from build123d import *

# Parameters (mm, degrees)
SKETCH1_R                = 150
BOSS_EXTRUDE1_DEPTH      = 75
CHAMFER1_SIZE            = 10
BOSS_EXTRUDE2_START      = -75
BOSS_EXTRUDE2_DEPTH      = 10
CHAMFER2_SIZE            = 10
BOSS_EXTRUDE3_DEPTH      = 10
BOSS_EXTRUDE4_DEPTH      = 3.5
CIRPATTERN1_COUNT        = 4
CIRPATTERN1_COPY_1_DEPTH = 10
CIRPATTERN1_COPY_2_DEPTH = 10
CIRPATTERN1_COPY_3_DEPTH = 10
CIRPATTERN1_COPY_4_DEPTH = 3.5
CIRPATTERN1_COPY_5_DEPTH = 3.5
CIRPATTERN1_COPY_6_DEPTH = 3.5
CUT_EXTRUDE1_START       = -50
CUT_EXTRUDE1_DEPTH       = 50
CIRPATTERN2_COUNT        = 4
SKETCH7_R                = 110
BOSS_EXTRUDE5_DEPTH      = 9
BOSS_EXTRUDE5_TAPER      = 45
SKETCH8_R                = 15
BOSS_EXTRUDE6_DEPTH      = 20
SKETCH9_W                = 52.192884268
SKETCH9_H                = 17.88463766
BOSS_EXTRUDE7_DEPTH      = 3
BOSS_EXTRUDE8_DEPTH      = 2


# Read off the part's stored shape, not the designer's step: Cut-Extrude1
with BuildPart() as part:
    # Sketch1 → Boss-Extrude1 (new body)
    with BuildSketch(Plane(origin=(0, 0, 0), x_dir=(1, 0, 0), z_dir=(0, 1, 0))):
        with Locations(Location((0, 0, 0), (0, 0, 270))):
            Circle(SKETCH1_R)
    extrude(amount=BOSS_EXTRUDE1_DEPTH)

    # Chamfer1
    chamfer1_edges = [part.edges().sort_by_distance(p)[0] for p in [
        (0, 75, -150),
    ]]
    chamfer(chamfer1_edges, length=CHAMFER1_SIZE)

    # Sketch3 → Boss-Extrude2 (add)
    with BuildSketch(Plane(origin=(0, 75, 0), x_dir=(1, 0, 0), z_dir=(0, 1, 0)).offset(BOSS_EXTRUDE2_START)):
        with BuildLine():
            Line((-145.236875483, 37.5), (-195.236875483, 37.5))
            Line((-195.236875483, 37.5), (-195.236875483, -37.5))
            Line((-195.236875483, -37.5), (-145.236875483, -37.5))
            ThreePointArc((-145.236875483, -37.5), (-150, 0), (-145.236875483, 37.5))
        make_face()
    boss_extrude2 = extrude(amount=BOSS_EXTRUDE2_DEPTH)

    # Chamfer2
    chamfer2_edges = [part.edges().sort_by_distance(p)[0] for p in [
        (-195.236875483, 5, -37.5),
        (-195.236875483, 5, 37.5),
    ]]
    chamfer(chamfer2_edges, length=CHAMFER2_SIZE)

    # Sketch4 → Boss-Extrude3 (add)
    with BuildSketch(Plane.XY.offset(37.5)):
        Polygon((-185.236875483, 10), (-145.236875483, 10), (-145.236875483, 65), (-168.236875483, 65), align=None)
    boss_extrude3 = extrude(amount=-BOSS_EXTRUDE3_DEPTH)

    # Sketch5 → Boss-Extrude4 (add)
    with BuildSketch(Plane(origin=(0, 10, 0), x_dir=(1, 0, 0), z_dir=(0, 1, 0))):
        Polygon((-185.236875483, -20), (-180.04072306, -17), (-180.04072306, -11), (-185.236875483, -8), (-190.433027905, -11), (-190.433027905, -17), align=None)
    boss_extrude4 = extrude(amount=BOSS_EXTRUDE4_DEPTH)

    # Mirror1: Boss-Extrude3, Boss-Extrude4 across plane
    add(boss_extrude3.mirror(Plane.XY))
    add(boss_extrude4.mirror(Plane.XY))

    # CirPattern1: Boss-Extrude2, Boss-Extrude3, Boss-Extrude4 ×4 about axis
    cirpattern1_axis = Axis((0, 0, 0), (0, 1, 0))
    add([boss_extrude2.rotate(cirpattern1_axis, i * 360 / CIRPATTERN1_COUNT) for i in range(1, CIRPATTERN1_COUNT)])
    add([boss_extrude3.rotate(cirpattern1_axis, i * 360 / CIRPATTERN1_COUNT) for i in range(1, CIRPATTERN1_COUNT)])
    add([boss_extrude4.rotate(cirpattern1_axis, i * 360 / CIRPATTERN1_COUNT) for i in range(1, CIRPATTERN1_COUNT)])

    # CirPattern1 copy 1 sketch → CirPattern1 copy 1 (add)
    with BuildSketch(Plane(origin=(-37.5, 0, 0), x_dir=(0, 0, -1), z_dir=(-1, 0, 0))):
        Polygon((-185.236875483, -10), (-145.236875483, -10), (-145.236875483, -65), (-168.236875483, -65), align=None)
    extrude(amount=-CIRPATTERN1_COPY_1_DEPTH)

    # CirPattern1 copy 2 sketch → CirPattern1 copy 2 (add)
    with BuildSketch(Plane(origin=(0, 0, 37.5), x_dir=(-1, 0, 0), z_dir=(0, 0, 1))):
        Polygon((-185.236875483, -10), (-145.236875483, -10), (-145.236875483, -65), (-168.236875483, -65), align=None)
    extrude(amount=-CIRPATTERN1_COPY_2_DEPTH)

    # CirPattern1 copy 3 sketch → CirPattern1 copy 3 (add)
    with BuildSketch(Plane(origin=(37.5, 0, 0), x_dir=(0, 0, 1), z_dir=(1, 0, 0))):
        Polygon((-185.236875483, -10), (-145.236875483, -10), (-145.236875483, -65), (-168.236875483, -65), align=None)
    extrude(amount=-CIRPATTERN1_COPY_3_DEPTH)

    # CirPattern1 copy 4 sketch → CirPattern1 copy 4 (add)
    with BuildSketch(Plane(origin=(0, 10, 0), x_dir=(0, 0, -1), z_dir=(0, 1, 0))):
        Polygon((-185.236875483, 20), (-180.04072306, 17), (-180.04072306, 11), (-185.236875483, 8), (-190.433027905, 11), (-190.433027905, 17), align=None)
    extrude(amount=CIRPATTERN1_COPY_4_DEPTH)

    # CirPattern1 copy 5 sketch → CirPattern1 copy 5 (add)
    with BuildSketch(Plane(origin=(0, 10, 0), x_dir=(-1, 0, 0), z_dir=(0, 1, 0))):
        Polygon((-185.236875483, 20), (-180.04072306, 17), (-180.04072306, 11), (-185.236875483, 8), (-190.433027905, 11), (-190.433027905, 17), align=None)
    extrude(amount=CIRPATTERN1_COPY_5_DEPTH)

    # CirPattern1 copy 6 sketch → CirPattern1 copy 6 (add)
    with BuildSketch(Plane.ZX.offset(10)):
        Polygon((-185.236875483, 20), (-180.04072306, 17), (-180.04072306, 11), (-185.236875483, 8), (-190.433027905, 11), (-190.433027905, 17), align=None)
    extrude(amount=CIRPATTERN1_COPY_6_DEPTH)

    # Cut-Extrude1 outline → Cut-Extrude1 (cut)
    with BuildSketch(Plane(origin=(0, 75, 0), x_dir=(1, 0, 0), z_dir=(0, 1, 0)).offset(CUT_EXTRUDE1_START)):
        with BuildLine():
            ThreePointArc((-65, -112.583302492), (-91.923881554, -91.923881554), (-112.583302492, -65))
            Line((-112.583302492, -65), (-129.903810568, -75))
            ThreePointArc((-129.903810568, -75), (-106.066017178, -106.066017178), (-75, -129.903810568))
            Line((-75, -129.903810568), (-65, -112.583302492))
        make_face()
    cut_extrude1 = extrude(amount=CUT_EXTRUDE1_DEPTH, mode=Mode.SUBTRACT)

    # CirPattern2: Cut-Extrude1 ×4 about axis
    cirpattern2_axis = Axis((1.096442134, 0, -1.096442134), (0, 1, 0))
    for i in range(1, CIRPATTERN2_COUNT):
        add(cut_extrude1.rotate(cirpattern2_axis, i * 360 / CIRPATTERN2_COUNT), mode=Mode.SUBTRACT)

    # Sketch7 → Boss-Extrude5 (add)
    with BuildSketch(Plane(origin=(0, 75, 0), x_dir=(1, 0, 0), z_dir=(0, 1, 0))):
        Circle(SKETCH7_R)
    extrude(amount=BOSS_EXTRUDE5_DEPTH, taper=BOSS_EXTRUDE5_TAPER)

    # Sketch8 → Boss-Extrude6 (add)
    with BuildSketch(Plane(origin=(0, 84, 0), x_dir=(1, 0, 0), z_dir=(0, 1, 0))):
        with Locations(Location((0, 0, 0), (0, 0, 270))):
            Circle(SKETCH8_R)
    extrude(amount=BOSS_EXTRUDE6_DEPTH)

    # Sketch9 → Boss-Extrude7 (add)
    with BuildSketch(Plane(origin=(0, 75, 0), x_dir=(1, 0, 0), z_dir=(0, 1, 0))):
        with Locations((1.096442134, -121.525621322)):
            Rectangle(SKETCH9_W, SKETCH9_H)
    extrude(amount=BOSS_EXTRUDE7_DEPTH)

    # Sketch10 → Boss-Extrude8 (add)
    with BuildSketch(Plane(origin=(0, 78, 0), x_dir=(1, 0, 0), z_dir=(0, 1, 0))):
        with BuildLine():
            Line((6.270682812, -126.545342988), (8.874678556, -128.884668308))
            Line((8.874678556, -128.884668308), (10.207504523, -127.401046891))
            Line((10.207504523, -127.401046891), (7.367027593, -124.84927636))
            ThreePointArc((7.367027593, -124.84927636), (-4.827336948, -118.169160855), (6.270682812, -126.545342988))
        make_face()
        with BuildLine():
            Line((4.310616526, -122.103519263), (2.977790559, -123.58714068))
            Line((2.977790559, -123.58714068), (4.010713475, -124.515077192))
            ThreePointArc((4.010713475, -124.515077192), (-2.528998008, -120.272284372), (4.900321371, -122.63328644))
            Line((4.900321371, -122.63328644), (4.310616526, -122.103519263))
        make_face(mode=Mode.SUBTRACT)
    extrude(amount=BOSS_EXTRUDE8_DEPTH)


solid = part.part
For this review, take the finished solid that the model builds, in its own axes (mm). A direction names the side the tool comes from. Coordinates: 2 decimals unless noted, no trailing zeros. Order: outer loops, then holes, each group sorted by start corner. A loop starts at its lowest first (then second) coordinate and runs counter-clockwise, first axis right, second up. Notation, with made-up numbers: (-35.75, -8) - (3.25, -8) arc R33 cw to (3.25, 24) - close; hole circle Ø3 at (18.5, -1.5). An arc over 180 degrees is marked (long way). Answer as CSV lines item,"result". Start each with the question number.
1) Insertion check: P1, Ø8, axis at x = 56.5, z = -34.5, coming from the +Y side; P2, Ø1, axis at x = 76.5, y = 57, coming from the -Z side; P3, Ø6, axis at y = 17.5, z = -124.5, coming from the +X side. Each pin has a flat end and moves straight along its axis. Give the tip position at first contact, or say it passes through.
2) Machinability: for faces 1 (the flat face through (185, 13.5, 14)), 2 (the flat face through (14, 13.5, 185)), 3 (the flat face through (-161, 33, -37.5)), 4 (the flat face through (33, 65, -157)), which of the approach directions +Z, -Z, +X, -X, +Y, -Y give a long, thin tool a straight path to every point of the face, cutting with its end or side? Answer none if there is none.
3) To check wall thickness, follow line 1 along Z through (x, y) = (10.5, 12); line 2 along Y through (x, z) = (-112.5, -78.5); line 3 along Z through (x, y) = (-153, 26.5). State the ranges of each line that lie inside material, in increasing order. Write a range as [from, to].
4) Add section B-B (y = 70). State the section outline as (x, z) points.
5) Add section A-A (z = 160). State the section outline as (x, y) points.
6) Draft analysis for pull direction Z (two halves, no side actions). For faces 5 (the flat face through (3, 0, -3)), 6 (the flat face through (71.85, 49.65, 120.65)), 7 (the cylindrical face through (-105.272, 24.823, -106.854)), state which applies: +Z half, -Z half, draft (parallel to the pull), parting line (faces both ways), or undercut.
Result:
1,P1,"y = 84"
1,P2,"z = -109.21"
1,P3,"x = 87.96"
2,face 1,"+X, +Y"
2,face 2,"+Z, +Y"
2,face 3,"-Z, -X, +Y, -Y"
2,face 4,"-Z, +X, +Y"
3,line 1,"[-189.57, -180.91], [-149.63, 149.63], [180.91, 189.57]"
3,line 2,"[0, 25]"
3,line 3,"[-37.5, -27.5], [27.5, 37.5]"
4,outline,"(-125.57, 72.5) arc R145 ccw to (-124.61, -74.14) - (-112.58, -67.19) arc R130 ccw to (-65, -114.78) - (-71.55, -126.12) arc R145 ccw to (73.19, -125.17) - (67.19, -114.78) arc R130 ccw to (114.78, -67.19) - (125.17, -73.19) arc R145 ccw to (126.12, 71.55) - (114.78, 65) arc R130 ccw to (67.19, 112.58) - (74.14, 124.61) arc R145 ccw to (-72.5, 125.57) - (-65, 112.58) arc R130 ccw to (-112.58, 65) - close"
5,outline,"(-37.5, 0) - (37.5, 0) - (37.5, 65) - (27.5, 65) - (27.5, 10) - (-27.5, 10) - (-27.5, 65) - (-37.5, 65) - close"
6,face 5,"draft"
6,face 6,"undercut"
6,face 7,"-Z half"
